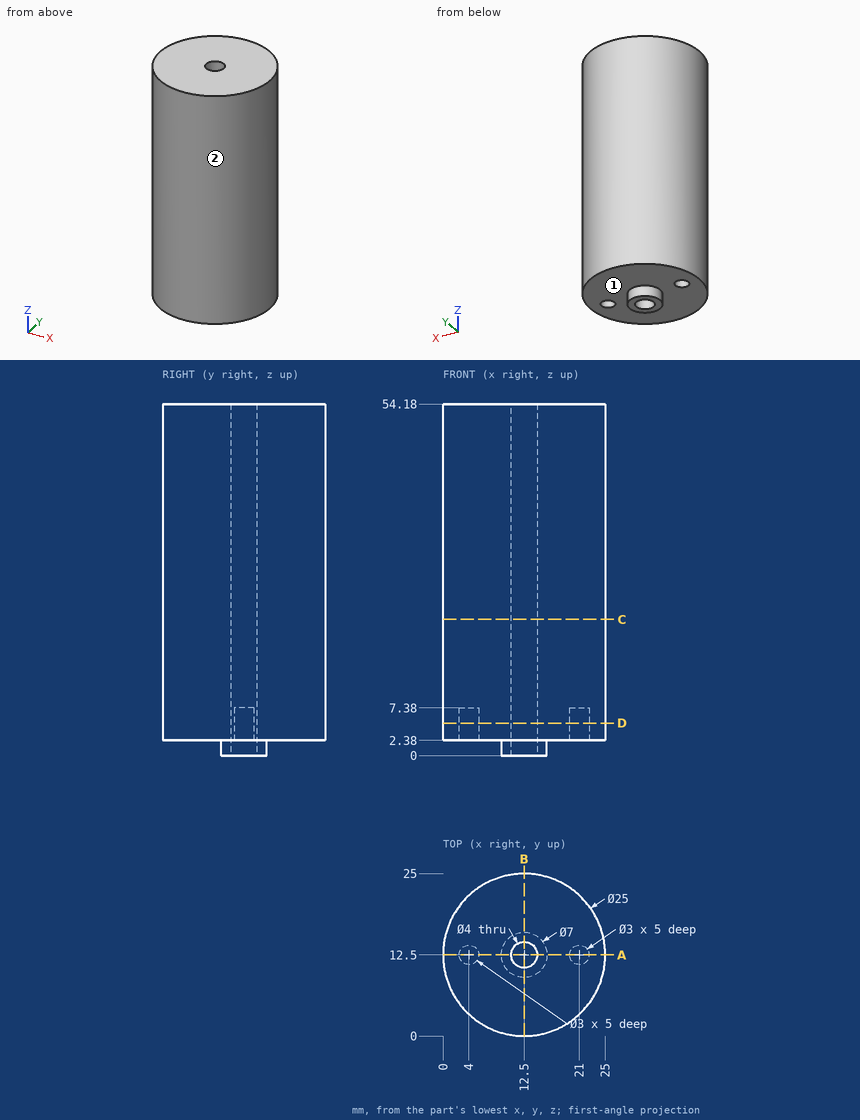
Part print with two shaded views. Sizes in mm from the minimum x, y, z corner. A direction names the side the tool comes from. Round coordinates to 2 decimals unless told otherwise and drop trailing zeros. Loops run counter-clockwise (first coordinate to the right, second up) from the corner with the lowest first, then second, coordinate; pieces in that order, holes last. Notation, with made-up numbers: (-2, 50.25) - (5, 50.25) arc R22 ccw to (5, 85.25) - close; hole circle Ø2 at (59, -8). An arc over 180 degrees is marked (long way). Answer as a JSON object with one key per item and string values.
Item 1: Band-saw the part on D-D on z = 5. List the corners of the cut face in (x, y).
Output:
{"outline": "circle Ø25 at (12.5, 12.5); hole circle Ø3 at (4, 12.5); hole circle Ø4 at (12.5, 12.5); hole circle Ø3 at (21, 12.5)"}
Item 2: Pin check, flat tips, straight feed: pin 1 (2 mm diameter, centred on x = 5.5, z = 9.5, fed in from -Y); pin 2 (5 mm diameter, centred on y = 3.5, z = 12.5, fed in from -X); pin 3 (3 mm diameter, centred on x = 20, z = 30.5, fed in from +Y). Stop position of each tip, or through.
Output:
{"pin 1": "y = 1.53", "pin 2": "x = 1.82", "pin 3": "y = 23.47"}
Item 3: Tool access for the marked faces 1 and 2: list every direction of +Z, -Z, +X, -X, +Y, -Y with a clear straight run to the whole face (end or side of a thin tool).
Output:
{"face 1": "-Z", "face 2": "+Z, -Z"}
Item 4: Band-saw the part on C-C on z = 21. List the corners of the cut face in (x, y).
Output:
{"outline": "circle Ø25 at (12.5, 12.5); hole circle Ø4 at (12.5, 12.5)"}
Item 5: Wall check: L1, parallel to Y at x = 12.5, z = 35.5; L2, parallel to Z at x = 6, y = 3.25; L3, parallel to Y at x = 21, z = 3.55. Give the ranges that are in metal, low to high.
Output:
{"L1": "0 to 10.5, 14.5 to 25", "L2": "2.38 to 54.18", "L3": "3.33 to 11, 14 to 21.67"}
Item 6: Band-saw the part on B-B on x = 12.5. List the corners of the cut face in (y, z), plus the area to 3 significant figures.
Output:
{"outline": "(0, 2.38) - (9, 2.38) - (9, 0) - (10.5, 0) - (10.5, 54.18) - (0, 54.18) - close; (14.5, 0) - (16, 0) - (16, 2.38) - (25, 2.38) - (25, 54.18) - (14.5, 54.18) - close", "area": "1,090 mm2"}
Item 7: Band-saw the part on A-A on y = 12.5. List the corners of the cut face in (x, z), plus the area to 3 significant figures.
Output:
{"outline": "(0, 2.38) - (2.5, 2.38) - (2.5, 7.38) - (5.5, 7.38) - (5.5, 2.38) - (9, 2.38) - (9, 0) - (10.5, 0) - (10.5, 54.18) - (0, 54.18) - close; (14.5, 0) - (16, 0) - (16, 2.38) - (19.5, 2.38) - (19.5, 7.38) - (22.5, 7.38) - (22.5, 2.38) - (25, 2.38) - (25, 54.18) - (14.5, 54.18) - close", "area": "1,060 mm2"}
